Part model, mm, in its own coordinate system. A direction names the side the tool comes from. Round coordinates to 2 decimals unless told otherwise and drop trailing zeros. Write each loop counter-clockwise with the first axis right and the second up, starting at its lowest first coordinate (ties: lowest second). Pieces come first, ordered by that corner, then holes. Notation, with made-up numbers: (-35, 42) -> (-17, 42) arc R29 ccw to (-17, 76) -> close; hole circle Ø1 at (33, 55.25). An arc over 180 degrees is marked (long way). Use CSV: the item, a comma, the result in double quotes. Start each with the question number.
(1) Saw through at A-A (x = 0). Give the cut face in (y, z), plus the area to 3 significant figures.
(2) Saw through at D-D (z = 8.5). Give the cut face in (x, y).
(3) Saw through at B-B (z = 0). Give the cut face in (x, y).
(4) Drop flat-ended pins along their axis: pin 1 (2 mm diameter, centred on x = -8, z = -3.5, fed in from +Y); pin 2 (2 mm diameter, centred on y = 2.5, z = -16, fed in from +X); pin 3 (3 mm diameter, centred on x = 1.5, y = 3, fed in from +Z). Give the stop position or say it passes through.
(5) Probe line 1 (Y direction, x = -16, z = -6.5). List the from-to ranges inside material, lowest first. Write a range as [from, to].
(6) Which spindle directions (+Z, -Z, +X, -X, +Y, -Y) get a long thin tool onto all of the face, cutting with end or side? Do faces 1 (the flat face through (0, -24, 21.15)), 2 (the cylindrical face through (-2.44, 11.83, -0.54)). Say none if no direction does.
(7) Saw through at C-C (y = 17.5). Give the cut face in (x, z), plus the area to 3 significant figures.
```python
from build123d import *

# Parameters (mm, degrees)
SKETCH2_R           = 2.5
BOSS_EXTRUDE1_DEPTH = 24
SKETCH1_W           = 42.3
SKETCH1_H           = 42.3
BOSS_EXTRUDE2_DEPTH = 48


with BuildPart() as part:
    # Sketch2 → Boss-Extrude1 (new body)
    with BuildSketch(Plane(origin=(0, 0, 0), x_dir=(1, 0, 0), z_dir=(0, 1, 0))):
        with Locations(Location((0, 0, 0), (0, 0, 270))):
            Circle(SKETCH2_R)
    extrude(amount=BOSS_EXTRUDE1_DEPTH)

    # Sketch1 → Boss-Extrude2 (add)
    with BuildSketch(Plane(origin=(0, 0, 0), x_dir=(1, 0, 0), z_dir=(0, 1, 0))):
        Rectangle(SKETCH1_W, SKETCH1_H)
    extrude(amount=-BOSS_EXTRUDE2_DEPTH)


solid = part.part
```
Answers:
1,outline,"(-48, -21.15) -> (0, -21.15) -> (0, -2.5) -> (24, -2.5) -> (24, 2.5) -> (0, 2.5) -> (0, 21.15) -> (-48, 21.15) -> close"
1,area,"2,150 mm²"
2,outline,"(-21.15, -48) -> (21.15, -48) -> (21.15, 0) -> (-21.15, 0) -> close"
3,outline,"(-21.15, -48) -> (21.15, -48) -> (21.15, 0) -> (2.5, 0) -> (2.5, 24) -> (-2.5, 24) -> (-2.5, 0) -> (-21.15, 0) -> close"
4,pin 1,"stops at y = 0"
4,pin 2,"passes through"
4,pin 3,"stops at z = 2.5"
5,line 1,"y = [-48, 0]"
6,face 1,"+Z, +X, -X, +Y, -Y"
6,face 2,"+Y"
7,outline,"circle Ø5 at (0, 0)"
7,area,"19.6 mm²"
